For this review, use the dimensioned drawing (mm, ordinates from the lowest corner) and the shaded views. A direction names the side the tool comes from. Coordinates: 2 decimals unless noted, no trailing zeros. Loops run counter-clockwise (first coordinate to the right, second up) from the corner with the lowest first, then second, coordinate; pieces in that order, holes last. Notation, with made-up numbers: (67, 78) - (111, 78) arc R7 ccw to (111, 86) - close; hole circle Ø10 at (72, 78). An arc over 180 degrees is marked (long way). Answer in a Markdown table with one row per item. Add a question column.
(1) The part is to be moulded in two halves that separate along Z. For the marked faces 1, 2 and 3, say which applies: released by +Z, released by -Z, zero draft, split by the parting line, or undercut.
(2) Clearance check with a flat-ended pin moving along its axis: pin 1 (10.5 mm diameter, centred on y = 37, z = 43, fed in from +X). State where the tip first meets the part, or that it passes through.
(3) We need section A-A, the plane x = 34. Write out the cut boundary in (y, z), plus the area to 3 significant figures.
(4) We need section B-B, the plane y = 51.5. Write out the cut boundary in (x, z).
(5) For the marked faces 4 and 5, list the 3-axis set-ups (+Z, -Z, +X, -X, +Y, -Y) from which the entire face can be reached by the end or side of a thin tool; tool diameter is ignored.
(6) To check wall thickness, follow L1, parallel to Z at x = 44, y = 51; L2, parallel to X at y = 59, z = 36. State the ranges of each line that lie inside material, in increasing order. Write a range as [from, to].
(7) We need section C-C, the plane z = 47. Write out the cut boundary in (x, y), plus the area to 4 significant figures.
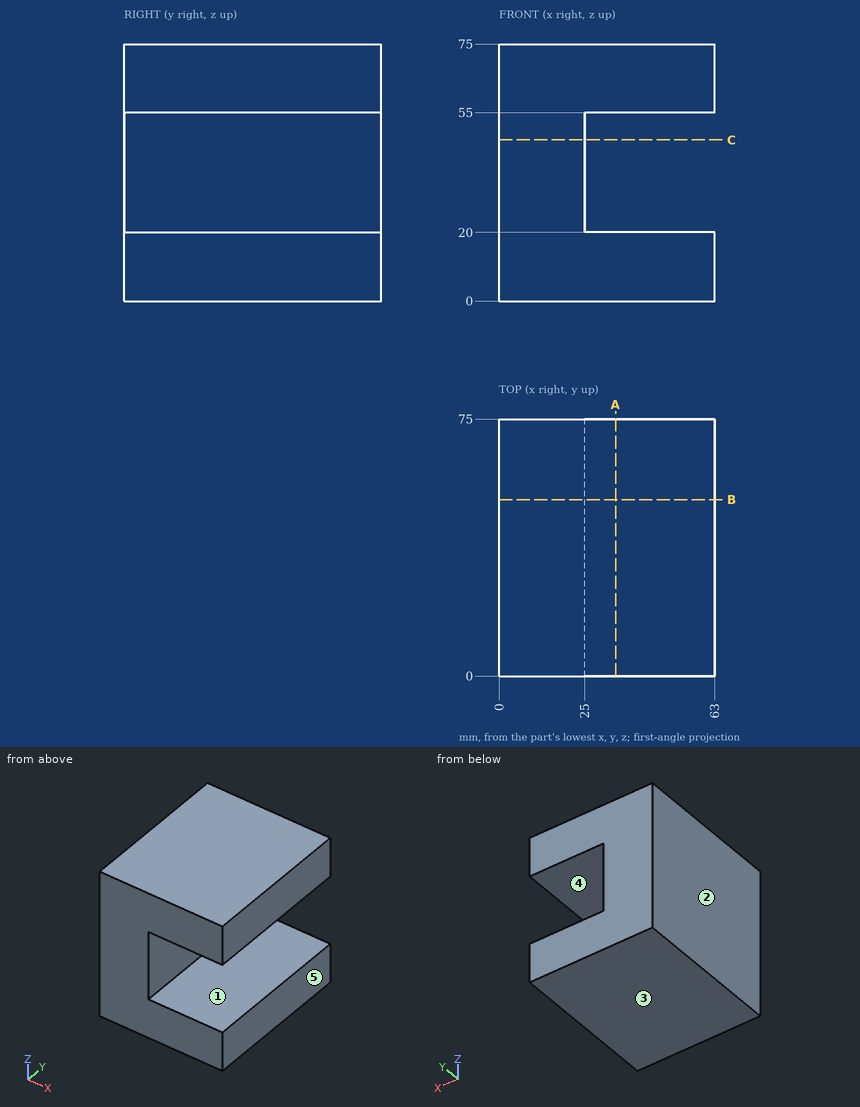
Responses:
| question | item | result |
|---|---|---|
| 1 | face 1 | undercut |
| 1 | face 2 | zero draft |
| 1 | face 3 | released by -Z |
| 2 | pin 1 | stops at x = 25 |
| 3 | outline | (0, 0) - (75, 0) - (75, 20) - (0, 20) - close; (0, 55) - (75, 55) - (75, 75) - (0, 75) - close |
| 3 | area | 3,000 mm2 |
| 4 | outline | (0, 0) - (63, 0) - (63, 20) - (25, 20) - (25, 55) - (63, 55) - (63, 75) - (0, 75) - close |
| 5 | face 4 | +X, +Y, -Y |
| 5 | face 5 | +Z, -Z, +X, +Y, -Y |
| 6 | L1 | z = [0, 20], [55, 75] |
| 6 | L2 | x = [0, 25] |
| 7 | outline | (0, 0) - (25, 0) - (25, 75) - (0, 75) - close |
| 7 | area | 1,875 mm2 |
